Source: CAD feature listing. Evaluate the final solid. Frame: model axes, mm. Round coordinates to 2 decimals unless told otherwise and drop trailing zeros. Write each loop counter-clockwise with the first axis right and the second up, starting at its lowest first coordinate (ties: lowest second). Pieces come first, ordered by that corner, then holes. Notation, with made-up numbers: M -36.5,40 L 10.5,40 A12 ccw 10.5,54 Z; hole C -21,71 d1. An arc over 180 degrees is marked long. Answer in a Markdown table with one row per item. Add a question column.
Item 1: Cut plane C-C on x = -4.5. Return loops of the section in (y, z), and give its area (3 significant figures).
Item 2: Cut plane A-A on x = 5. Return loops of the section in (y, z).
Item 3: Contact query for flat-ended pins moving along their axis: pin 1 (1 mm diameter, centred on x = 7, z = 2, fed in from -Y); pin 2 (1.5 mm diameter, centred on y = -17, z = 4.5, fed in from +X). Output: stop coordinate, or through.
Item 4: Mould query, pull axis X, two halves, no side actions, for faces 1 (the face through (23.824, 1.914, 3.451)), 2 (the face through (-32.702, -12.352, 3.451)), 3 (the face through (16.332, -3.806, 3.451)). Classes: released by +X, released by -X, zero draft, split by the parting line, or undercut.
Item 5: Cut plane B-B on y = 0. Return loops of the section in (x, z), and give its area (3 significant figures).
Item 6: Cut plane D-D on z = 3.5. Return loops of the section in (x, y).
Item 7: Material intervals for probe 1 along Y at (x, z) = (-4, 1.5); probe 2 along X at (y, z) = (-17.5, 3.25); probe 3 along X at (y, z) = (9, 5.5), sorted ascending.
from build123d import *

# Parameters (mm, degrees)
F0_R     = 6.75
F0_R_2   = 11
F1_DEPTH = 7


with BuildPart() as f1:
    # F0 (on Top) → F1 (new body)
    with BuildSketch(Plane.XY):
        with BuildLine():
            ThreePointArc((0.0303634628, 34.8677483042), (-4.1124282103, 33.9830527199), (-7.5172278162, 31.4625867377))
            ThreePointArc((-7.5172278162, 31.4625867377), (-13.6121821661, 19.4898899069), (-13.2411988753, 6.0602097422))
            ThreePointArc((-13.2411988753, 6.0602097422), (-22.9967779432, -1.7556709932), (-34.2936443309, -7.1073178834))
            ThreePointArc((-34.2936443309, -7.1073178834), (-32.6733499934, -12.4241997031), (-30.2115375356, -17.407578622))
            ThreePointArc((-30.2115375356, -17.407578622), (-27.3739728485, -20.5529936613), (-23.4887854755, -22.2414036237))
            ThreePointArc((-23.4887854755, -22.2414036237), (-10.0726486933, -21.5334405102), (1.3723038486, -14.4973194736))
            ThreePointArc((1.3723038486, -14.4973194736), (13.0188446523, -19.0379584074), (23.3019400052, -26.1455082372))
            ThreePointArc((23.3019400052, -26.1455082372), (27.0963475613, -22.0838512694), (30.1811740728, -17.4601696823))
            ThreePointArc((30.1811740728, -17.4601696823), (31.4864010588, -13.4300590586), (31.0060132917, -9.221183114))
            ThreePointArc((31.0060132917, -9.221183114), (23.6848308594, 2.0435506033), (11.8688950266, 8.4371097315))
            ThreePointArc((11.8688950266, 8.4371097315), (9.9779332908, 20.7936294005), (10.9917043257, 33.2528261205))
            ThreePointArc((10.9917043257, 33.2528261205), (5.5770024321, 34.5080509726), (0.0303634628, 34.8677483042))
        make_face()
        with Locations((-21.5361416876, -12.4338972007)):
            Circle(F0_R, mode=Mode.SUBTRACT)
        with BuildLine():
            ThreePointArc((-12.6630806003, -17.045706709), (-11.4611852349, -12.169559613), (-12.5478578488, -7.2664477846))
            ThreePointArc((-12.5478578488, -7.2664477846), (-9.5228828701, -10.9345645475), (-5.47403134, -13.4270242753))
            ThreePointArc((-5.47403134, -13.4270242753), (-8.7901592188, -15.7894419215), (-12.6630806003, -17.045706709))
        make_face(mode=Mode.SUBTRACT)
        with BuildLine():
            ThreePointArc((1.4389157248, -14.428427549), (1.4056400908, -14.4629028124), (1.3723038486, -14.4973194736))
            ThreePointArc((1.3723038486, -14.4973194736), (1.2826311608, -14.4740053694), (1.1929184258, -14.4508458448))
            ThreePointArc((1.1929184258, -14.4508458448), (1.3159648149, -14.4401605464), (1.4389157248, -14.428427549))
        make_face(mode=Mode.SUBTRACT)
        with Locations((21.5361416876, -12.4338972007)):
            Circle(F0_R, mode=Mode.SUBTRACT)
        Circle(F0_R_2, mode=Mode.SUBTRACT)
        with BuildLine():
            ThreePointArc((14.3651597896, 1.9728619361), (18.069137425, 0.282219774), (21.0935553356, -2.4436961356))
            ThreePointArc((21.0935553356, -2.4436961356), (16.2697403952, -3.8408977644), (12.5668573011, -7.2335397678))
            ThreePointArc((12.5668573011, -7.2335397678), (14.2310521125, -2.779776209), (14.3651597896, 1.9728619361))
        make_face(mode=Mode.SUBTRACT)
        with BuildLine():
            ThreePointArc((-8.4304747353, 19.4894028445), (-4.8085551602, 16.0104573774), (-0.0189994523, 14.4999875524))
            ThreePointArc((-0.0189994523, 14.4999875524), (-4.7081692424, 13.7143407565), (-8.8911284496, 11.4541623392))
            ThreePointArc((-8.8911284496, 11.4541623392), (-9.2789782062, 15.5072221475), (-8.4304747353, 19.4894028445))
        make_face(mode=Mode.SUBTRACT)
        with Locations((0, 24.8677944013)):
            Circle(F0_R, mode=Mode.SUBTRACT)
        with BuildLine():
            ThreePointArc((1.1929184258, -14.4508458448), (1.2826311608, -14.4740053694), (1.3723038486, -14.4973194736))
            ThreePointArc((1.3723038486, -14.4973194736), (1.4056400908, -14.4629028124), (1.4389157248, -14.428427549))
            ThreePointArc((1.4389157248, -14.428427549), (1.3159648149, -14.4401605464), (1.1929184258, -14.4508458448))
        make_face()
    extrude(amount=F1_DEPTH)


solid = f1.part
Results below:
| question | item | result |
|---|---|---|
| 1 | outline | M -19.09,0 L -10.04,0 L -10.04,7 L -19.09,7 Z; M 10.04,0 L 13.78,0 L 13.78,7 L 10.04,7 Z; M 15.83,0 L 19.84,0 L 19.84,7 L 15.83,7 Z; M 29.9,0 L 33.8,0 L 33.8,7 L 29.9,7 Z |
| 1 | area | 145 mm2 |
| 2 | outline | M -15.58,0 L -9.8,0 L -9.8,7 L -15.58,7 Z; M 9.8,0 L 20.33,0 L 20.33,7 L 9.8,7 Z; M 29.4,0 L 34.59,0 L 34.59,7 L 29.4,7 Z |
| 3 | pin 1 | y = -16.5 |
| 3 | pin 2 | x = 30.78 |
| 4 | face 1 | released by +X |
| 4 | face 2 | released by -X |
| 4 | face 3 | undercut |
| 5 | outline | M -20.37,0 L -11,0 L -11,7 L -20.37,7 Z; M 11,0 L 14.5,0 L 14.5,7 L 11,7 Z; M 18.48,0 L 25.68,0 L 25.68,7 L 18.48,7 Z |
| 5 | area | 140 mm2 |
| 6 | outline | M -34.29,-7.11 A34.13 ccw -30.21,-17.41 A10 ccw -23.49,-22.24 A27.23 ccw 1.37,-14.5 A53.76 cw 23.3,-26.15 A34.13 ccw 30.18,-17.46 A10 ccw 31.01,-9.22 A27.23 ccw 11.87,8.44 A53.76 cw 10.99,33.25 A34.13 ccw 0.03,34.87 A10 ccw -7.52,31.46 A27.23 ccw -13.24,6.06 A53.76 cw Z; hole C -21.54,-12.43 d13.5; hole M -12.66,-17.05 A13.39 ccw -5.47,-13.43 A14.5 cw -12.55,-7.27 A11.02 cw Z; hole C 0,0 d22; hole M -8.89,11.45 A14.5 cw -0.02,14.5 A11.02 cw -8.43,19.49 A13.39 ccw Z; hole C 0,24.87 d13.5; hole M 12.57,-7.23 A11.02 cw 21.09,-2.44 A13.39 ccw 14.37,1.97 A14.5 cw Z; hole C 21.54,-12.43 d13.5 |
| 7 | probe 1 | -18.79 to -10.25, 10.25 to 13.94, 15.58 to 19.43, 30.3 to 34.03 |
| 7 | probe 2 | -30.16 to -26, -17.08 to -2.08, 9.88 to 17.08, 26 to 30.16 |
| 7 | probe 3 | -13.9 to -6.32, 6.32 to 11.72 |
